Geometry: see drawing. Coordinates: mm, zero at the bounding-box minimum. A direction names the side the tool comes from. Give positions to 0.01 mm unless a question says otherwise; leave off trailing zeros. Write each loop counter-clockwise with the first axis right and the second up, starting at its lowest first coordinate (ties: lowest second). Pieces come first, ordered by that corner, then holes.
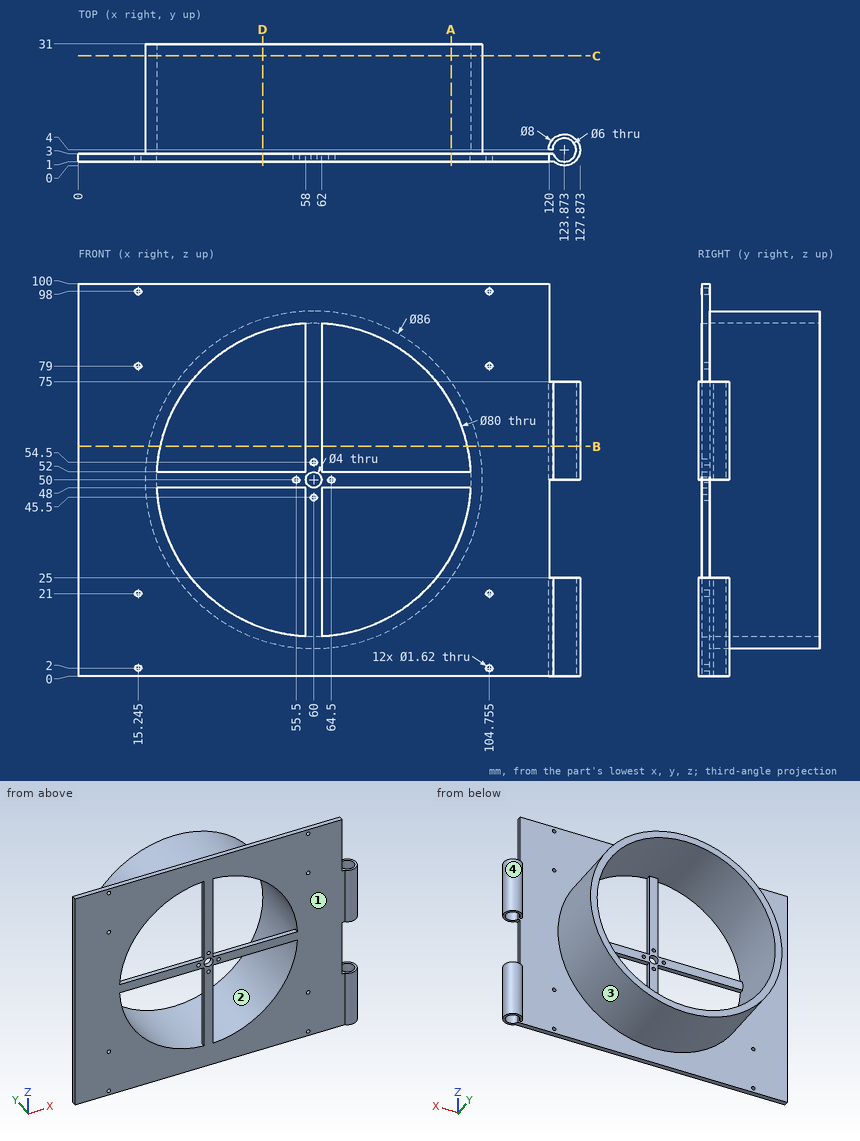
1. Section query D-D (x = 47). Return loops of the section in (y, z), plus the area to 3 significant figures.
2. Pull-direction query (X, two-part tool) for the marked faces 1 and 2; classes: pulls with the +X half, pulls with the -X half, needs draft (parallel to the pull), parting line crosses it, or undercut.
3. Section query B-B (z = 58.5). Return loops of the section in (x, y).
4. Access query for the marked faces 3 and 4. Directions: +Z, -Z, +X, -X, +Y, -Y. A direction counts if a zero-diameter tool reaches every point of the face in a straight line with its end or side. Return the directions, or none.
5. Pin query (flat end, axial travel): P1, Ø2, axis at y = 7, z = 47, coming from the -X side; P2, Ø3.5, axis at x = 60, z = 50, coming from the +Y side; P3, Ø2, axis at y = 6.5, z = 72.5, coming from the -X side; P4, Ø1.1, axis at x = 120.5, z = 12.5, coming from the -Y side. Return the tip coordinate at first contact, or that it passes through.
6. Section query C-C (y = 28). Return loops of the section in (x, z).
7. Section query A-A (x = 95). Return loops of the section in (y, z).
8. Line query: probe 1 along Z at (x, y) = (61, 19); probe 2 along Y at (x, z) = (20, 91); probe 3 along Z at (x, y) = (78, 28). Output: solid intervals per line, ascending.
The answers:
1. outline: (1, 0) - (3, 0) - (3, 9.01) - (31, 9.01) - (31, 12.17) - (1, 12.17) - close; (1, 48) - (3, 48) - (3, 52) - (1, 52) - close; (1, 87.83) - (31, 87.83) - (31, 90.99) - (3, 90.99) - (3, 100) - (1, 100) - close
1. area: 234 mm2
2. face 1: needs draft
2. face 2: undercut
3. outline: (0, 1) - (20.91, 1) - (20.91, 31) - (17.85, 31) - (17.85, 3) - (0, 3) - close; (58, 1) - (62, 1) - (62, 3) - (58, 3) - close; (99.09, 1) - (121.23, 1) arc R4 ccw (long way) to (119.87, 4) - (120.87, 4) arc R3 cw (long way) to (121.04, 3) - (102.15, 3) - (102.15, 31) - (99.09, 31) - close
4. face 3: +Y
4. face 4: +Z, -Z
5. P1: stops at x = 17.05
5. P2: passes through
5. P3: stops at x = 22.76
5. P4: stops at y = 1
6. outline: circle Ø86 at (60, 50); hole circle Ø80 at (60, 50)
7. outline: (1, 0) - (3, 0) - (3, 25.02) - (31, 25.02) - (31, 30.64) - (1, 30.64) - close; (1, 48) - (3, 48) - (3, 52) - (1, 52) - close; (1, 69.36) - (31, 69.36) - (31, 74.98) - (3, 74.98) - (3, 100) - (1, 100) - close
8. probe 1: z = 7.01 to 10.01, 89.99 to 92.99
8. probe 2: y = 1 to 3
8. probe 3: z = 10.95 to 14.28, 85.72 to 89.05
